Design review of the part built by this model. Coordinates are the model's own, in mm. A direction names the side the tool comes from. Coordinates: 2 decimals unless noted, no trailing zeros. Write each loop counter-clockwise with the first axis right and the second up, starting at its lowest first coordinate (ties: lowest second). Pieces come first, ordered by that corner, then holes.
Q1. For L1, parallel to Z at x = -79, y = -44; L2, parallel to Z at x = 90.5, y = -92; L3, parallel to X at y = 38, z = 34, list the stretches that pass through material, from the lowest coordinate up.
Q2. The part is to be moulded in two halves that separate along Z. For faces 1 (the flat face through (103.124, -1, 21)), 2 (the conical face through (166.22, -0.64, 101.21)), 3 (the flat face through (-93, 1, 43.18)), say which applies: released by +Z, released by -Z, zero draft, split by the parting line, or undercut.
Q3. Take a section at C-C, the plane z = 184.5. Write out the cut boundary in (x, y) (3 decimals), plus the area to 3 significant figures.
Q4. For faces 4 (the flat face through (-1, -23.562, 185)), 5 (the flat face through (71, -52.07, 117)), 6 (the flat face through (71, 52.07, 117)), list the 3-axis set-ups (+Z, -Z, +X, -X, +Y, -Y) from which the entire face can be reached by the end or side of a thin tool; tool diameter is ignored.
Q5. Take a section at B-B, the plane z = 27. Write out the cut boundary in (x, y) (3 decimals), plus the area to 3 significant figures.
Q6. Take a section at D-D, the plane x = 133. Write out the cut boundary in (y, z) (3 decimals), plus the area to 3 significant figures.
Q7. Take a section at A-A, the plane x = 0. Write out the cut boundary in (y, z) (3 decimals), plus the area to 3 significant figures.
Q8. For pin 1 Ø2.5 at (x, z) = (-147, 131) entering from +Y; pin 2 Ø4 at (y, z) = (68, 102.5) entering from -X; pin 3 Ø17 at (x, z) = (78.5, 123.5) entering from -Y, all flat-tipped, find the tip position at first contact; note any pin that passes through.
from build123d import *

# Parameters (mm, degrees)
SKETCH1_W           = 206.248
SKETCH1_H           = 206.248
C_DIM_DEPTH         = 43.18
SHAFT_START         = 12.7
SKETCH_A_R          = 15.875
SHAFT_DEPTH         = 153.67
SKETCH3_W           = 104.14
SKETCH3_H           = 104.14
BOSS_EXTRUDE3_DEPTH = 99.568
FILLET1_R           = 5.715
FILLET4_R           = 5.715
SKETCH4_R           = 77.597
BOSS_EXTRUDE4_DEPTH = 133.35
BOSS_EXTRUDE4_TAPER = 5
FILLET2_R           = 8.255
SKETCH5_W           = 99.328405226
SKETCH5_H           = 47.124202614
BOSS_EXTRUDE5_DEPTH = 20.32
CHAMFER1_SIZE       = 0.381
FILLET3_R           = 3.175
CUT_EXTRUDE_START   = 12.3698
CUT_EXTRUDE_B_DEPTH = 68.6402


with BuildPart() as part:
    # Sketch1 → C dim (new body)
    with BuildSketch(Plane.XY):
        Rectangle(SKETCH1_W, SKETCH1_H)
    extrude(amount=C_DIM_DEPTH)



with BuildPart() as body_2:
    # Sketch A → Shaft (new body)
    with BuildSketch(Plane(origin=(0, 0, 0), x_dir=(0, 0, -1), z_dir=(1, 0, 0)).offset(SHAFT_START)):
        with Locations((-116.84, 0)):
            Circle(SKETCH_A_R)
    extrude(amount=SHAFT_DEPTH)

    # Chamfer1
    chamfer1_edges = [body_2.edges().sort_by_distance(p)[0] for p in [
        (166.37, 0, 132.715),
    ]]
    chamfer(chamfer1_edges, length=CHAMFER1_SIZE)

    # Sketch6 → Cut-Extrude B (cut, through all)
    with BuildSketch(Plane.XY.offset(116.84).offset(CUT_EXTRUDE_START)):
        with BuildLine():
            Line((166.37, -3.175), (109.093, -3.175))
            ThreePointArc((109.093, -3.175), (105.918, 0), (109.093, 3.175))
            Line((109.093, 3.175), (166.37, 3.175))
            ThreePointArc((166.37, 3.175), (169.545, 0), (166.37, -3.175))
        make_face()
    extrude(amount=CUT_EXTRUDE_B_DEPTH, mode=Mode.SUBTRACT)


with BuildPart() as body_3:
    # Sketch3 → Boss-Extrude3 (new body)
    with BuildSketch(Plane(origin=(0, 0, 0), x_dir=(0, 0, -1), z_dir=(1, 0, 0))):
        with Locations((-116.84, 0)):
            Rectangle(SKETCH3_W, SKETCH3_H)
    extrude(amount=BOSS_EXTRUDE3_DEPTH)


with BuildPart() as body_4:
    # Mirror2: mirrored copy
    add(body_3.part.mirror(Plane(origin=(0, 0, 0), x_dir=(0, 0, 1), z_dir=(1, 0, 0))))

    # Fillet4
    fillet4_edges = [body_4.edges().sort_by_distance(p)[0] for p in [
        (-49.784, 52.07, 64.77),
        (-49.784, 52.07, 168.91),
        (-49.784, -52.07, 168.91),
        (-49.784, -52.07, 64.77),
    ]]
    fillet(fillet4_edges, radius=FILLET4_R)


with BuildPart() as body_3_1:
    add(body_3.part)

    # Fillet1
    fillet1_edges = [body_3_1.edges().sort_by_distance(p)[0] for p in [
        (49.784, 52.07, 64.77),
        (49.784, 52.07, 168.91),
        (49.784, -52.07, 168.91),
        (49.784, -52.07, 64.77),
    ]]
    fillet(fillet1_edges, radius=FILLET1_R)


with BuildPart() as part_1:
    add(part.part)

    add(body_3_1.part)  # Boss-Extrude4 merges body 3

    add(body_4.part)  # Boss-Extrude4 merges body 4
    # Sketch4 → Boss-Extrude4 (add)
    with BuildSketch(Plane.XY.offset(43.18)):
        Circle(SKETCH4_R)
    extrude(amount=BOSS_EXTRUDE4_DEPTH, taper=BOSS_EXTRUDE4_TAPER)

    # Fillet2
    fillet2_edges = [part_1.edges().sort_by_distance(p)[0] for p in [
        (-65.930386719, 0, 176.53),
        (-77.597, 0, 43.18),
        (-103.124, 103.124, 21.59),
        (103.124, 103.124, 21.59),
        (103.124, -103.124, 21.59),
        (-103.124, -103.124, 21.59),
    ]]
    fillet(fillet2_edges, radius=FILLET2_R)

    # Sketch5 → Boss-Extrude5 (add)
    with BuildSketch(Plane.XY.offset(176.53)):
        Rectangle(SKETCH5_W, SKETCH5_H)
    extrude(amount=BOSS_EXTRUDE5_DEPTH)

    # Fillet3
    fillet3_edges = [part_1.edges().sort_by_distance(p)[0] for p in [
        (-49.664202613, 23.562101307, 186.69),
        (-49.664202613, -23.562101307, 186.69),
        (49.664202613, -23.562101307, 186.69),
        (49.664202613, 23.562101307, 186.69),
        (0, 23.562101307, 196.85),
        (-49.664202613, 0, 196.85),
        (0, -23.562101307, 196.85),
        (49.664202613, 0, 196.85),
    ]]
    fillet(fillet3_edges, radius=FILLET3_R)


with BuildPart() as body_3_2:
    # Mirror6: mirrored copy
    add(body_2.part.mirror(Plane(origin=(0, 0, 0), x_dir=(0, 0, 1), z_dir=(1, 0, 0))))


with BuildPart() as part_2:
    add(part_1.part)

    # Combine1: union body 2, body 3 2
    add(body_2.part)
    add(body_3_2.part)


solid = part_2.part
Responses:
1. L1: z = 0 to 43.18, 64.77 to 168.91
1. L2: z = 0 to 43.18
1. L3: x = -103.12 to 103.12
2. face 1: zero draft
2. face 2: split by the parting line
2. face 3: undercut
3. outline: (-49.664, -20.387) arc R3.175 ccw to (-46.489, -23.562) - (46.489, -23.562) arc R3.175 ccw to (49.664, -20.387) - (49.664, 20.387) arc R3.175 ccw to (46.489, 23.562) - (-46.489, 23.562) arc R3.175 ccw to (-49.664, 20.387) - close
3. area: 4,670 mm2
4. face 4: +Z, +X, -X, -Y
4. face 5: +Z, +X, -Y
4. face 6: +Z, +X, +Y
5. outline: (-103.124, -94.869) arc R8.255 ccw to (-94.869, -103.124) - (94.869, -103.124) arc R8.255 ccw to (103.124, -94.869) - (103.124, 94.869) arc R8.255 ccw to (94.869, 103.124) - (-94.869, 103.124) arc R8.255 ccw to (-103.124, 94.869) - close
5. area: 42,500 mm2
6. outline: (-3.175, 129.21) - (-3.175, 132.394) arc R15.875 ccw (long way) to (3.175, 132.394) - (3.175, 129.21) - close
6. area: 770 mm2
7. outline: (-103.124, 0) - (103.124, 0) - (103.124, 43.18) - (85.161, 43.18) arc R8.255 cw to (76.938, 50.716) - (66.59, 168.994) arc R8.255 ccw to (58.366, 176.53) - (23.562, 176.53) - (23.562, 193.675) arc R3.175 ccw to (20.387, 196.85) - (-20.387, 196.85) arc R3.175 ccw to (-23.562, 193.675) - (-23.562, 176.53) - (-58.366, 176.53) arc R8.255 ccw to (-66.59, 168.994) - (-76.938, 50.716) arc R8.255 cw to (-85.161, 43.18) - (-103.124, 43.18) - close
7. area: 29,000 mm2
8. pin 1: stops at y = 9.24
8. pin 2: stops at x = -29.8
8. pin 3: stops at y = -52.07
